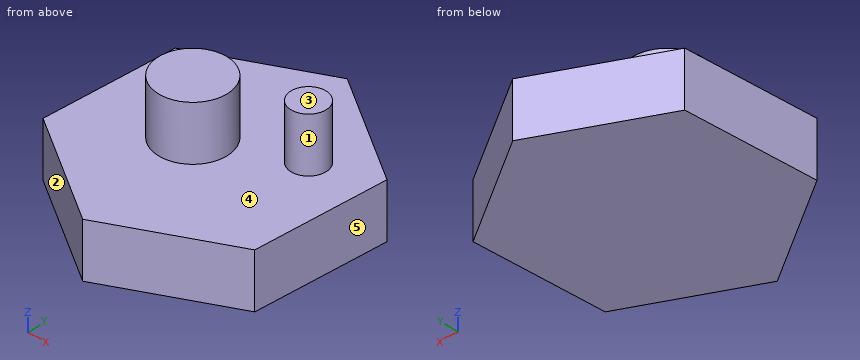
from build123d import *

# Parameters (mm, degrees)
F1_DEPTH = 25
F2_R     = 15.578145
F3_DEPTH = 25
F4_R     = 7.947035
F5_DEPTH = 25


with BuildPart() as f1:
    # F0 (on Top) → F1 (new body)
    with BuildSketch(Plane.XY):
        Polygon((4.813501, 59.28203), (-48.932993, 33.809629), (-53.746495, -25.472401), (-4.813501, -59.28203), (48.932993, -33.809629), (53.746495, 25.472401), align=None)
    extrude(amount=F1_DEPTH)

    # F2 (on face) → F3 (join)
    with BuildSketch(Plane.XY.offset(25)):
        with Locations((-9.968227, 0)):
            Circle(F2_R)
    extrude(amount=F3_DEPTH)

    # F4 (on face) → F5 (join)
    with BuildSketch(Plane.XY.offset(25)):
        with Locations((27.919721, 15.267807)):
            Circle(F4_R)
    extrude(amount=F5_DEPTH)


solid = f1.part
Can you work these out from the model? Positions are in its coordinate system, mm. Face numbers are marked on the shaded views. A direction names the side the tool comes from. Coordinates: 2 decimals unless noted, no trailing zeros. Write each loop counter-clockwise with the first axis right and the second up, starting at its lowest first coordinate (ties: lowest second). Pieces come first, ordered by that corner, then holes. Notation, with made-up numbers: (-20.5, 14) - (1.5, 14) arc R25 cw to (1.5, 27) - close; hole circle Ø2 at (63.5, 18.25). An arc over 180 degrees is marked (long way). Return JSON: item names as keys, results as strings. Group by question number.
Item 1: I'm going to push flat-ended pins straight in: pin 1 Ø1 at (y, z) = (6, 39.5) entering from -X; pin 2 Ø2 at (x, z) = (16, 5.5) entering from +Y; pin 3 Ø2 at (x, y) = (18.5, 13.5) entering from +Z. Where does each tip first touch, or does it pass through?
Item 2: We'd pull the mould along X, two halves only. Please class the marked faces 1, 2 and 3: pulls with the +X half, pulls with the -X half, needs draft (parallel to the pull), parting line crosses it, or undercut.
Item 3: If we section it at B-B (x = 33): Write out the boundary of the cut face in (y, z).
Item 4: Please list where these lines run through material, in increasing order: probe 1 along Z at (x, y) = (-6, 36); probe 2 along X at (y, z) = (1, 20); probe 3 along X at (y, z) = (-6, 12.5).
Item 5: If we section it at A-A (y = -5.5): Write out the boundary of the cut face in (x, z), then the cut area to 3 significant figures.
Item 6: Which directions (+Z, -Z, +X, -X, +Y, -Y) give clear straight access to the entire face, cutting with the end or side of a thin tool? Please do the marked faces 4 and 5.
Item 7: If we section it at C-C (z = 20): Write out the boundary of the cut face in (x, y).
Item 8: If we section it at D-D (z = 47.5): Write out the boundary of the cut face in (x, y), then the cut area to 3 significant figures.
Return value:
{
 "1": {"pin 1": "stops at x = -24.54", "pin 2": "stops at y = 52.24", "pin 3": "stops at z = 25"},
 "2": {"face 1": "undercut", "face 2": "pulls with the -X half", "face 3": "needs draft"},
 "3": {"outline": "(-41.36, 0) - (39.81, 0) - (39.81, 25) - (21.38, 25) - (21.38, 50) - (9.16, 50) - (9.16, 25) - (-41.36, 25) - close"},
 "4": {"probe 1": "z = 0 to 25", "probe 2": "x = -51.6 to 51.76", "probe 3": "x = -52.17 to 51.19"},
 "5": {"outline": "(-52.12, 0) - (51.23, 0) - (51.23, 25) - (4.61, 25) - (4.61, 50) - (-24.54, 50) - (-24.54, 25) - (-52.12, 25) - close", "area": "3,310 mm^2"},
 "6": {"face 4": "+Z", "face 5": "+Z, -Z, +X, -Y"},
 "7": {"outline": "(-53.75, -25.47) - (-4.81, -59.28) - (48.93, -33.81) - (53.75, 25.47) - (4.81, 59.28) - (-48.93, 33.81) - close"},
 "8": {"outline": "circle Ø31.16 at (-9.97, 0); circle Ø15.89 at (27.92, 15.27)", "area": "961 mm^2"}
}
